Autodesk Inventor part; units mm, degrees
ref_plane "YZ Plane" through (0, 0, 0) normal (1, 0, 0) x (0, 1, 0)
ref_plane "XZ Plane" through (0, 0, 0) normal (0, 1, 0) x (-1, 0, 0)
ref_plane "XY Plane" through (0, 0, 0) normal (0, 0, 1) x (1, 0, 0)
sketch "Pulley Sketch" plane through (0, 0, 0) normal (0, 0, 1) x (1, 0, 0)
  circle A0 centre (0, 0) radius 15.1595 construction
  circle A1 centre (0, 0) radius 14.7785
  circle A2 centre (0, 0) radius 12.1115
  line L0 (-2.422, 14.5787) -> (-1.524, 12.1115)
  line L1 (-1.524, 12.1115) -> (1.524, 12.1115)
  line L2 (1.524, 12.1115) -> (2.422, 14.5787)
  line L3 (0, 0) -> (0, 14.7785) construction
  point P0 (0, 12.1115)
  dimension "d0" = 30.319
  dimension "d1" = 0.381
  dimension "d2" = 2.667
  dimension "d3" = 40
  dimension "d4" = 3.048
extrude "Base Body" add sketch "Pulley Sketch" along normal mid plane 12 contours A2 | A1 L0 L1 L2 | L2 L1 L0 A1
extrude "Tooth" cut sketch "Pulley Sketch" along normal through all both and the other way through all contours L2 L1 L0 A1 picked at (0, 13.8747)
fillet "Tooth Fillet" radius 1.1938 2 edges at (1.524, 12.1115, 0) (-1.524, 12.1115, 0)
fillet "Tooth Fillet" radius 1.1684 4 edges at (-2.422, 14.5787, 3) (-2.422, 14.5787, -3) (2.422, 14.5787, 3) (2.422, 14.5787, -3)
pattern_circular "Teeth" count 10 over 360 about axis through (0, 0, -10) along (0, 0, 1) of "Tooth", "Tooth Fillet"
feature "Left flange" [suppressed]
feature "Right flange" [suppressed]
sketch "Sketch2" plane through (0, 0, 6) normal (0, 0, 1) x (1, 0, 0)
  circle A0 centre (0, 0) radius 7.5
  dimension "d17" = 15
extrude "Extrusion3" cut sketch "Sketch2" against normal through all
equation "\"d1\" = da_a"
equation "\"d2\" = da_hg"
equation "\"d3\" = 2 * da_fi"
equation "\"d4\" = da_bw"
equation "\"d5\" = da_bf"
equation "\"d7\" = da_bf"
equation "\"d9\" = da_rb"
equation "\"d10\" = da_rt"
equation "\"da_pb\" = 9.525"
equation "\"da_fi\" = 20deg"
equation "\"da_hg\" = 2.667"
equation "\"da_bw\" = 3.048"
equation "\"da_rb\" = 1.1938"
equation "\"da_rt\" = 1.1684"
equation "\"da_a\" = 0.381"
equation "\"da_bf\" = 12"
equation "\"da_wf\" = 1.5"
equation "\"da_hf\" = 1.5"
properties part number "Synchronous Pulley1" material "Steel"
Build history of the part. All positions in model axes, mm. A direction names the side the tool comes from. Coordinates: 2 decimals unless noted, no trailing zeros. Order: outer loops, then holes, each group sorted by start corner. A loop starts at its lowest first (then second) coordinate and runs counter-clockwise, first axis right, second up. Notation, with made-up numbers: (80.5, 30.25) -> (89.5, 30.25) arc R24 cw to (89.5, 53.25) -> close; hole circle Ø7 at (-11.5, 86.25). An arc over 180 degrees is marked (long way). Answer in a Markdown table with one row per item. Add a question column.
Q1. Band-saw the part on A-A, the plane x = 0. List the corners of the cut face in (y, z), then the cut area to 3 significant figures.
Q2. Mould opens along X. For faces 1 (the face through (10.5, -10, 0.1)), 2 (the face through (-11.3, 5.12, -0.08)), 3 (the face through (4.55, -14.06, 0.08)) say: +X half, -X half, draft (parallel to the pull), parting line (faces both ways), or undercut.
Q3. Wall check: line 1 along Y through (x, z) = (0, 2.25); line 2 along X through (y, z) = (9.5, -2); line 3 along X through (y, z) = (6.5, 4.5). Give the ranges that are in metal, low to high. Write a range as [from, to].
Q4. Band-saw the part on B-B, the plane y = 0. List the corners of the cut face in (x, z).
Q5. Which spindle directions (+Z, -Z, +X, -X, +Y, -Y) get a long thin tool onto all of the face, cutting with end or side? Do faces 4 (the face through (11.522, -3.733, -0.084)), 5 (the face through (1.381, 12.333, -0.084)), 6 (the face through (-7.111, -9.804, -0.084)). Say none if no direction does.
Q6. Drop flat-ended pins along their axis: pin 1 (1.1 mm diameter, centred on x = 0, z = 1.5, fed in from +Y); pin 2 (4 mm diameter, centred on y = 6.5, z = 0.5, fed in from +X); pin 3 (0.7 mm diameter, centred on x = 0, z = 0, fed in from -Y). Give the stop position or say it passes through.
Answers follow:
| question | item | result |
|---|---|---|
| 1 | outline | (-12.11, -6) -> (-7.5, -6) -> (-7.5, 6) -> (-12.11, 6) -> close; (7.5, -6) -> (12.11, -6) -> (12.11, 6) -> (7.5, 6) -> close |
| 1 | area | 111 mm^2 |
| 2 | face 1 | undercut |
| 2 | face 2 | -X half |
| 2 | face 3 | +X half |
| 3 | line 1 | [-12.11, -7.5], [7.5, 12.11] |
| 3 | line 2 | [-11.32, -9.24], [-7.53, 7.53], [9.24, 11.32] |
| 3 | line 3 | [-12.6, -3.74], [3.74, 12.6] |
| 4 | outline | (-14.78, -6) -> (-7.5, -6) -> (-7.5, 6) -> (-14.78, 6) -> close; (7.5, -6) -> (14.78, -6) -> (14.78, 6) -> (7.5, 6) -> close |
| 5 | face 4 | +Z, -Z, +X |
| 5 | face 5 | +Z, -Z, +Y |
| 5 | face 6 | +Z, -Z, -Y |
| 6 | pin 1 | y = 12.11 |
| 6 | pin 2 | x = 12.77 |
| 6 | pin 3 | y = -12.11 |
